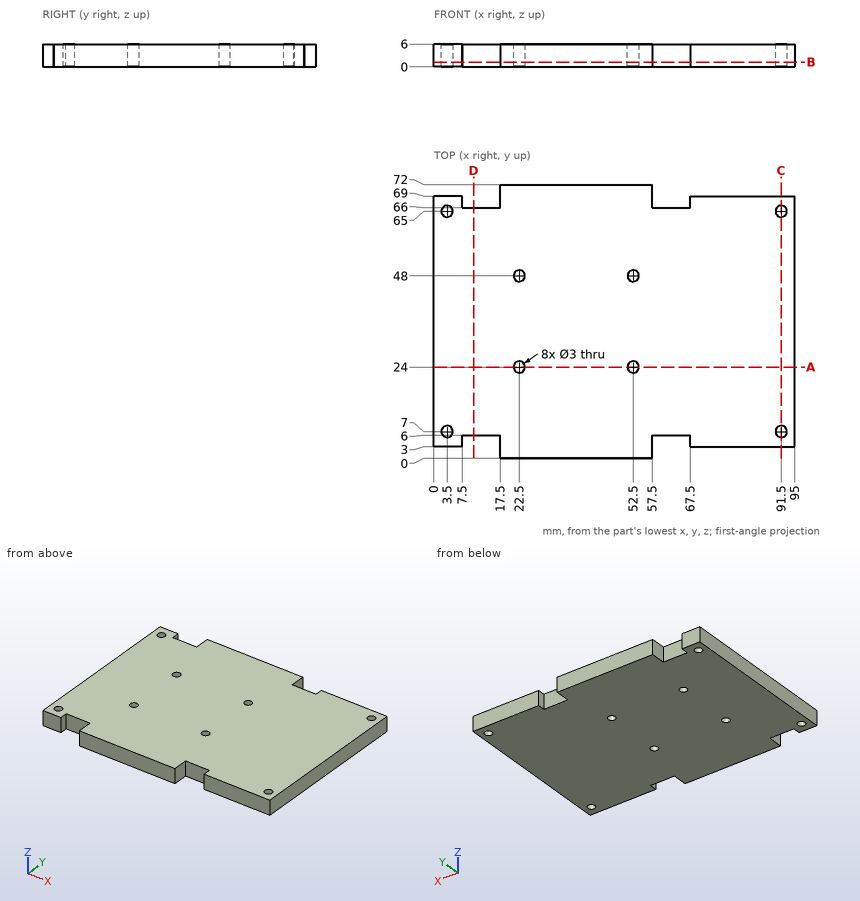
Design review of the part shown in the three views and the two pictorial views. Dimensions are in mm from the part's minimum x, y and z. Give positions to 0.01 mm unless a question says otherwise; leave off trailing zeros. Loops run counter-clockwise (first coordinate to the right, second up) from the corner with the lowest first, then second, coordinate; pieces in that order, holes last. Notation, with made-up numbers: M 24.25,-31.5 L 31.25,-31.5 A27 ccw 31.25,-2.5 Z; hole C 6.25,-8.5 d1. An arc over 180 degrees is marked long. Put each result on its own line as item: value. Start each with the question number.
(1) Add section A-A, the plane y = 24. Write out the cut boundary in (x, z), then the cut area to 3 significant figures.
(2) Wall thickness on L1, parallel to X at y = 65, z = 1.75; L2, parallel to Y at x = 52.5, z = 2.1; L3, parallel to Y at x = 3.5, z = 4.7: over which ranges is each line inside the solid? List them lowest first.
(3) Add section D-D, the plane x = 10.5. Write out the cut boundary in (y, z).
(4) Add section B-B, the plane z = 1.2. Give the number of separate pieces and of enclosed holes in the cut face, then the cut area to 3 significant figures.
(5) Add section C-C, the plane x = 91.5. Write out the cut boundary in (y, z).
(6) For pin 1 (2 mm diameter, centred on x = 74, z = 5, fed in from +Y); pin 2 (1.8 mm diameter, centred on x = 63, z = 2, fed in from +Y); pin 3 (3 mm diameter, centred on x = 65.5, z = 0.5, fed in from -Y); pin 4 (2.5 mm diameter, centred on x = 3.5, y = 7, fed in from +Z), all flat-tipped, find the tip position at first contact; note any pin that passes through.
Result:
1. outline: M 0,0 L 21,0 L 21,6 L 0,6 Z; M 24,0 L 51,0 L 51,6 L 24,6 Z; M 54,0 L 95,0 L 95,6 L 54,6 Z
1. area: 534 mm^2
2. L1: x = 0 to 2, 5 to 90, 93 to 95
2. L2: y = 0 to 22.5, 25.5 to 46.5, 49.5 to 72
2. L3: y = 3 to 5.5, 8.5 to 63.5, 66.5 to 69
3. outline: M 6,0 L 66,0 L 66,6 L 6,6 Z
4. separate pieces: 1
4. enclosed holes: 8
4. area: 6,330 mm^2
5. outline: M 3,0 L 5.5,0 L 5.5,6 L 3,6 Z; M 8.5,0 L 63.5,0 L 63.5,6 L 8.5,6 Z; M 66.5,0 L 69,0 L 69,6 L 66.5,6 Z
6. pin 1: stops at y = 69
6. pin 2: stops at y = 66
6. pin 3: stops at y = 6
6. pin 4: passes through
